Design review of the part built by this model. Coordinates are the model's own, in mm. Face numbers are marked on the shaded views. A direction names the side the tool comes from. Coordinates: 2 decimals unless noted, no trailing zeros. Loops run counter-clockwise (first coordinate to the right, second up) from the corner with the lowest first, then second, coordinate; pieces in that order, holes last. Notation, with made-up numbers: (22.5, 66.25) - (79.5, 66.25) arc R14 ccw to (79.5, 77.25) - close; hole circle Ø8 at (-25, 40.5). An arc over 180 degrees is marked (long way). Return JSON: item names as keys, results as strings. Group by question number.
from build123d import *

# Parameters (mm, degrees)
BOSS_EXTRUDE1_DEPTH = 22.0218
SKETCH3_R           = 5.9944
BOSS_EXTRUDE2_DEPTH = 11.0236
SKETCH4_R           = 3.0226
CUT_EXTRUDE1_DEPTH  = 12.5476
SKETCH5_R           = 1.27
CUT_EXTRUDE2_DEPTH  = 6.35


with BuildPart() as part:
    # Sketch1 → Boss-Extrude1 (new body)
    with BuildSketch(Plane.XY):
        Polygon((2.302357403, 3.9878), (-2.302357403, 3.9878), (-4.604714807, 0), (-2.302357403, -3.9878), (2.302357403, -3.9878), (4.604714807, 0), align=None)
    extrude(amount=-BOSS_EXTRUDE1_DEPTH)

    # Sketch3 → Boss-Extrude2 (add)
    with BuildSketch(Plane(origin=(0, 0, -22.0218), x_dir=(-1, 0, 0), z_dir=(0, 0, -1))):
        Circle(SKETCH3_R)
    extrude(amount=BOSS_EXTRUDE2_DEPTH)

    # Sketch4 → Cut-Extrude1 (cut)
    with BuildSketch(Plane(origin=(0, 0, -33.0454), x_dir=(-1, 0, 0), z_dir=(0, 0, -1))):
        Circle(SKETCH4_R)
    extrude(amount=-CUT_EXTRUDE1_DEPTH, mode=Mode.SUBTRACT)

    # Sketch5 → Cut-Extrude2 (cut)
    with BuildSketch(Plane(origin=(-5.19130268, -2.9972, 0), x_dir=(0, 0, 1), z_dir=(-0.8660254037844376, -0.500000000000002, 0))):
        with Locations(Location((-29.2354, 0, 0), (0, 0, 270))):
            Circle(SKETCH5_R)
    extrude(amount=-CUT_EXTRUDE2_DEPTH, mode=Mode.SUBTRACT)


solid = part.part
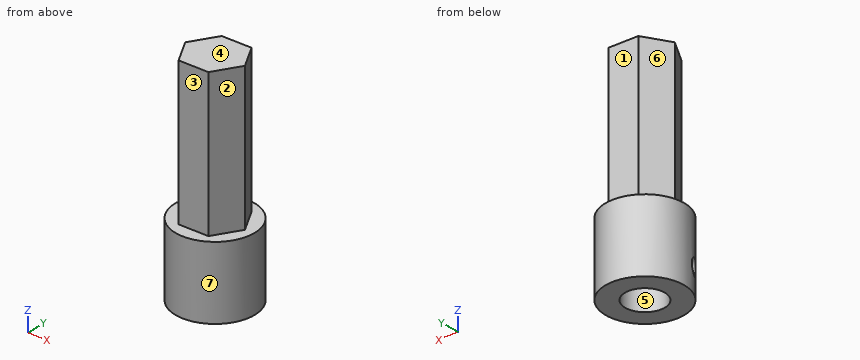
Item 1: Add section C-C (y = 2.25). State the section outline as (x, z) points.
Item 2: Add section B-B (x = 0). State the section outline as (y, z) points, then the cut area to 3 significant figures.
Item 3: Draft analysis for pull direction X (two halves, no side actions). For the marked faces 5, 6 and 7, state which applies: pulls with the +X half, pulls with the -X half, needs draft (parallel to the pull), parting line crosses it, or undercut.
Item 4: Add section D-D (x = 3.5). State the section outline as (y, z) points.
Item 5: For the marked faces 1, 2, 3 and 4, list the 3-axis set-ups (+Z, -Z, +X, -X, +Y, -Y) from which the entire face can be reached by the end or side of a thin tool; tool diameter is ignored.
Item 6: For P1, Ø1.4, axis at x = 0, z = -9.5, coming from the +Y side; P2, Ø6, axis at x = -4, z = -9.5, coming from the -Y side; P3, Ø1.5, axis at y = 3.5, z = -10, coming from the +X side, all flat-tipped, find the tip position at first contact; note any pin that passes through.
Item 7: To check wall thickness, follow line 1 (Y direction, x = 0, z = -25.5); line 2 (Z direction, x = 1.5, y = 2.5); line 3 (Z direction, x = -5, y = 3). State the ranges of each line that lie inside material, in increasing order. Write a range as from..to.
Item 8: Add section A-A (z = -3.5). State the section outline as (x, y) points.
Answers below:
{
 "1": {"outline": "(-5.56, -33.05) - (-2.02, -33.05) - (-2.02, -20.5) - (2.02, -20.5) - (2.02, -33.05) - (5.56, -33.05) - (5.56, -22.02) - (3.31, -22.02) - (3.31, 0) - (-3.31, 0) - (-3.31, -22.02) - (-5.56, -22.02) - close"},
 "2": {"outline": "(-5.99, -33.05) - (-3.02, -33.05) - (-3.02, -20.5) - (3.02, -20.5) - (3.02, -33.05) - (5.99, -33.05) - (5.99, -22.02) - (3.99, -22.02) - (3.99, 0) - (-3.99, 0) - (-3.99, -22.02) - (-5.99, -22.02) - close", "area": "232 mm^2"},
 "3": {"face 5": "undercut", "face 6": "pulls with the -X half", "face 7": "parting line crosses it"},
 "4": {"outline": "(-4.87, -33.05) - (4.87, -33.05) - (4.87, -22.02) - (1.91, -22.02) - (1.91, 0) - (-1.91, 0) - (-1.91, -22.02) - (-4.87, -22.02) - close"},
 "5": {"face 1": "+Z, +X, -X, +Y", "face 2": "+Z, +X, -Y", "face 3": "+Z, +X, -X, -Y", "face 4": "+Z, +X, -X, +Y, -Y"},
 "6": {"P1": "stops at y = 3.99", "P2": "stops at y = -3.99", "P3": "stops at x = 3.02"},
 "7": {"line 1": "y = -5.99..-3.02, 3.02..5.99", "line 2": "z = -20.5..0", "line 3": "z = -33.05..-22.02"},
 "8": {"outline": "(-4.6, 0) - (-2.3, -3.99) - (2.3, -3.99) - (4.6, 0) - (2.3, 3.99) - (-2.3, 3.99) - close"}
}
